The model under review builds one solid part; all positions refer to its coordinate system, in mm. Round coordinates to 2 decimals unless told otherwise and drop trailing zeros. Write each loop counter-clockwise with the first axis right and the second up, starting at its lowest first coordinate (ties: lowest second). Pieces come first, ordered by that corner, then holes. Notation, with made-up numbers: (-25.75, 12.5) -> (15.25, 12.5) arc R17 ccw to (15.25, 24.5) -> close; hole circle Ø2 at (76.5, -39.75). An arc over 180 degrees is marked (long way). Use CSV: the item, a comma, the result in double quotes. Start each with the question number.
1) For pin 1 Ø10.5 at (x, y) = (99.5, 12.5) entering from +Z; pin 2 Ø1 at (x, z) = (21.5, -581) entering from +Y; pin 3 Ø3 at (y, z) = (5.5, -662.5) entering from -X; pin 4 Ø6.5 at (x, z) = (96, -125.2) entering from +Y, all flat-tipped, find the tip position at first contact; note any pin that passes through.
2) Take a section at C-C, the plane y = 12.5. Give the boundary of the cut face in (x, z), then the cut area to 3 significant figures.
3) Take a section at B-B, the plane x = 23. Give the boundary of the cut face in (y, z), then the cut area to 3 significant figures.
4) Wall thickness on probe 1 along X at (y, z) = (18.8, -797.2); probe 2 along Y at (x, z) = (96.5, -524.5); probe 3 along Y at (x, z) = (59.5, -592): over which ranges is each line inside the solid? List them lowest first. Write a range as [from, to].
5) Take a section at A-A, the plane z = -760. Give the boundary of the cut face in (x, y), then the cut area to 3 significant figures.
6) Mouldability with a two-part tool opening along Y and no side actions: class faces 1 (the face through (102, 9, -457)), 2 (the face through (50, -1, -459)), 3 (the face through (55.1, -0.7, -905.2)) as released by +Y, released by -Y, zero draft, split by the parting line, or undercut.
from build123d import *

# Parameters (mm, degrees)
SKETCH1_W                    = 103
SKETCH1_H                    = 905.2
BASE_FLANGE1_DEPTH           = 1
EDGE_FLANGE1_STRIP_W         = 6
EDGE_FLANGE1_STRIP_H         = 1
EDGE_FLANGE1_STRIP_CUT_DEPTH = 905.2
EDGE_FLANGE1_DEPTH           = 905.2
EDGE_FLANGE2_STRIP_W         = 6
EDGE_FLANGE2_STRIP_H         = 1
EDGE_FLANGE2_STRIP_CUT_DEPTH = 905.2
EDGE_FLANGE2_DEPTH           = 905.2
SKETCH19_R                   = 2.5
CUT_EXTRUDE2_DEPTH           = 10
CUT_EXTRUDE3_START           = -20.5
CUT_EXTRUDE3_DEPTH           = 20.5


# Read off the part's stored shape, not the designer's step: Cut-Extrude3
# Sheet-metal steps are written as plain solids
with BuildPart() as part:
    # Sketch1 → Base-Flange1 (new body)
    with BuildSketch(Plane(origin=(0, 0, 0), x_dir=(1, 0, 0), z_dir=(0, 1, 0))):
        with Locations((51.5, 452.6)):
            Rectangle(SKETCH1_W, SKETCH1_H)
    extrude(amount=-BASE_FLANGE1_DEPTH)

    # Edge-Flange1 strip (across the edge) → Edge-Flange1 strip cut (cut)
    with BuildSketch(Plane(origin=(103, 0, 0), x_dir=(-1, 0, 0), z_dir=(0, 0, -1))):
        with Locations((-1, -0.5)):
            Rectangle(EDGE_FLANGE1_STRIP_W, EDGE_FLANGE1_STRIP_H)
    extrude(amount=EDGE_FLANGE1_STRIP_CUT_DEPTH, mode=Mode.SUBTRACT)

    # Edge-Flange1 section (across the edge) → Edge-Flange1 (add)
    with BuildSketch(Plane(origin=(103, 0, 0), x_dir=(-1, 0, 0), z_dir=(0, 0, -1))):
        with BuildLine():
            Line((0, 1), (0, 19))
            Line((0, 19), (1, 19))
            Line((1, 19), (1, 1))
            ThreePointArc((1, 1), (1.292893219, 0.292893219), (2, 0))
            Line((2, 0), (2, -1))
            ThreePointArc((2, -1), (0.585786438, -0.414213562), (0, 1))
        make_face()
    extrude(amount=EDGE_FLANGE1_DEPTH)

    # Edge-Flange2 strip (across the edge) → Edge-Flange2 strip cut (cut)
    with BuildSketch(Plane(origin=(102, 19, 0), x_dir=(0, -1, 0), z_dir=(0, 0, -1))):
        with Locations((-1, -0.5)):
            Rectangle(EDGE_FLANGE2_STRIP_W, EDGE_FLANGE2_STRIP_H)
    extrude(amount=EDGE_FLANGE2_STRIP_CUT_DEPTH, mode=Mode.SUBTRACT)

    # Edge-Flange2 section (across the edge) → Edge-Flange2 (add)
    with BuildSketch(Plane(origin=(102, 19, 0), x_dir=(0, -1, 0), z_dir=(0, 0, -1))):
        with BuildLine():
            Line((0, 1), (0, 12))
            Line((0, 12), (1, 12))
            Line((1, 12), (1, 1))
            ThreePointArc((1, 1), (1.292893219, 0.292893219), (2, 0))
            Line((2, 0), (2, -1))
            ThreePointArc((2, -1), (0.585786438, -0.414213562), (0, 1))
        make_face()
    extrude(amount=EDGE_FLANGE2_DEPTH)

    # Sketch19 → Cut-Extrude2 (cut)
    with BuildSketch(Plane(origin=(0, 19, 0), x_dir=(1, 0, 0), z_dir=(0, 1, 0))):
        with Locations(Location((96, 842.2, 0), (0, 0, 180))):
            Circle(SKETCH19_R)
        with Locations(Location((96, 797.2, 0), (0, 0, 180))):
            Circle(SKETCH19_R)
        with Locations(Location((96, 629.2, 0), (0, 0, 180))):
            Circle(SKETCH19_R)
        with Locations(Location((96, 461.2, 0), (0, 0, 180))):
            Circle(SKETCH19_R)
        with Locations(Location((96, 293.2, 0), (0, 0, 180))):
            Circle(SKETCH19_R)
        with Locations(Location((96, 125.2, 0), (0, 0, 180))):
            Circle(SKETCH19_R)
    extrude(amount=-CUT_EXTRUDE2_DEPTH, mode=Mode.SUBTRACT)

    # Cut-Extrude3 outline → Cut-Extrude3 (cut)
    with BuildSketch(Plane.XY.offset(CUT_EXTRUDE3_START)):
        with BuildLine():
            ThreePointArc((102, 1), (101.707106781, 0.292893219), (101, 0))
            Line((101, 0), (101, -1))
            ThreePointArc((101, -1), (102.414213562, -0.414213562), (103, 1))
            Line((103, 1), (103, 17))
            ThreePointArc((103, 17), (102.414213562, 18.414213562), (101, 19))
            Line((101, 19), (90, 19))
            Line((90, 19), (90, 18))
            Line((90, 18), (101, 18))
            ThreePointArc((101, 18), (101.707106781, 17.707106781), (102, 17))
            Line((102, 17), (102, 1))
        make_face()
    extrude(amount=CUT_EXTRUDE3_DEPTH, mode=Mode.SUBTRACT)


solid = part.part
Values found:
1,pin 1,"z = -20.5"
1,pin 2,"y = 0"
1,pin 3,"x = 102"
1,pin 4,"y = 19"
2,outline,"(102, -905.2) -> (103, -905.2) -> (103, -20.5) -> (102, -20.5) -> close"
2,area,"885 mm²"
3,outline,"(-1, -905.2) -> (0, -905.2) -> (0, 0) -> (-1, 0) -> close"
3,area,"905 mm²"
4,probe 1,"[90, 93.5], [98.5, 101.87]"
4,probe 2,"[-1, 0], [18, 19]"
4,probe 3,"[-1, 0]"
5,outline,"(0, -1) -> (101, -1) arc R2 ccw to (103, 1) -> (103, 17) arc R2 ccw to (101, 19) -> (90, 19) -> (90, 18) -> (101, 18) arc R1 cw to (102, 17) -> (102, 1) arc R1 cw to (101, 0) -> (0, 0) -> close"
5,area,"133 mm²"
6,face 1,"undercut"
6,face 2,"released by -Y"
6,face 3,"zero draft"
